from build123d import *

# Parameters (mm, degrees)
F1_DEPTH = 3.05


with BuildPart() as f1:
    # F0 (on Top) → F1 (new body, symmetric)
    with BuildSketch(Plane.XY):
        with BuildLine():
            ThreePointArc((13.3630401454, 32.8485820591), (9.568174531, 29.8987076881), (4.8777587712, 28.8485820591))
            Line((4.8777587712, 28.8485820591), (-45.1222412288, 28.8485820591))
            ThreePointArc((-45.1222412288, 28.8485820591), (-49.8126569886, 29.8987076881), (-53.6075226031, 32.8485820591))
            Line((-53.6075226031, 32.8485820591), (-71.3722412288, 32.8485820591))
            Line((-71.3722412288, 32.8485820591), (-71.3722412288, 14.8485820591))
            Line((-71.3722412288, 14.8485820591), (-53.6075226031, 14.8485820591))
            ThreePointArc((-53.6075226031, 14.8485820591), (-49.8126569886, 17.7984564302), (-45.1222412288, 18.8485820591))
            Line((-45.1222412288, 18.8485820591), (4.8777587712, 18.8485820591))
            ThreePointArc((4.8777587712, 18.8485820591), (9.568174531, 17.7984564302), (13.3630401454, 14.8485820591))
            Line((13.3630401454, 14.8485820591), (31.1277587712, 14.8485820591))
            Line((31.1277587712, 14.8485820591), (31.1277587712, 32.8485820591))
            Line((31.1277587712, 32.8485820591), (13.3630401454, 32.8485820591))
        make_face()
    extrude(amount=F1_DEPTH, both=True)


solid = f1.part
For this review, take the finished solid that the model builds, in its own axes (mm). A direction names the side the tool comes from. Coordinates: 2 decimals unless noted, no trailing zeros. Loops run counter-clockwise (first coordinate to the right, second up) from the corner with the lowest first, then second, coordinate; pieces in that order, holes last. Notation, with made-up numbers: (28.5, 19) - (71.5, 19) arc R15 cw to (71.5, 43) - close; hole circle Ø10 at (-5, 27.25). An arc over 180 degrees is marked (long way). Use a Markdown table: item, result. Add a question column.
Item 1: Insertion check: pin 1 Ø2 at (x, z) = (3.5, 2) entering from -Y. The pin has a flat end and moves straight along its axis. Give the tip position at first contact, or say it passes through.
Item 2: We need section D-D (x = 7). Give the boundary of the cut face in (y, z).
Item 3: Tool access review of faces 4 (the face through (-62, 32.849, 0)), 5 (the face through (-49.87, 17.77, 0.04)), 6 (the face through (9.63, 29.93, 0.04)): name each direction out of +Z, -Z, +X, -X, +Y, -Y from which nothing blocks a thin tool from reaching the whole face with its end or side.
Item 4: We need section B-B (y = 31.25). Give the boundary of the cut face in (x, z).
Item 5: We need section C-C (x = -5). Give the boundary of the cut face in (y, z).
Item 6: For line 1 (Y direction, x = -5, z = 0.5); line 2 (X direction, y = 17, z = 0.5); line 3 (X direction, y = 30, z = 0), list the stretches that pass through material, from the lowest coordinate up.
Item 7: Mouldability with a two-part tool opening along X and no side actions: class faces 1 (the face through (9.507, 17.827, 0.043)), 2 (the face through (31.128, 24, 0)), 3 (the face through (-71.372, 24, 0)) as pulls with the +X half, pulls with the -X half, needs draft (parallel to the pull), parting line crosses it, or undercut.
Item 8: We need section A-A (z = 0.75). Give the boundary of the cut face in (x, y), and give its area (3 significant figures).
Results list:
| question | item | result |
|---|---|---|
| 1 | pin 1 | stops at y = 18.85 |
| 2 | outline | (18.64, -3.05) - (29.06, -3.05) - (29.06, 3.05) - (18.64, 3.05) - close |
| 3 | face 4 | +Z, -Z, +X, -X, +Y |
| 3 | face 5 | +Z, -Z, -Y |
| 3 | face 6 | +Z, -Z, +Y |
| 4 | outline | (-71.37, -3.05) - (-51.98, -3.05) - (-51.98, 3.05) - (-71.37, 3.05) - close; (11.74, -3.05) - (31.13, -3.05) - (31.13, 3.05) - (11.74, 3.05) - close |
| 5 | outline | (18.85, -3.05) - (28.85, -3.05) - (28.85, 3.05) - (18.85, 3.05) - close |
| 6 | line 1 | y = 18.85 to 28.85 |
| 6 | line 2 | x = -71.37 to -51.23, 10.98 to 31.13 |
| 6 | line 3 | x = -71.37 to -50.02, 9.78 to 31.13 |
| 7 | face 1 | undercut |
| 7 | face 2 | pulls with the +X half |
| 7 | face 3 | pulls with the -X half |
| 8 | outline | (-71.37, 14.85) - (-53.61, 14.85) arc R11 cw to (-45.12, 18.85) - (4.88, 18.85) arc R11 cw to (13.36, 14.85) - (31.13, 14.85) - (31.13, 32.85) - (13.36, 32.85) arc R11 cw to (4.88, 28.85) - (-45.12, 28.85) arc R11 cw to (-53.61, 32.85) - (-71.37, 32.85) - close |
| 8 | area | 1,350 mm^2 |
